Source: CAD feature listing. Evaluate the final solid. Frame: model axes, mm. Coordinates: 2 decimals unless noted, no trailing zeros. Order: outer loops, then holes, each group sorted by start corner. A loop starts at its lowest first (then second) coordinate and runs counter-clockwise, first axis right, second up.
```python
from build123d import *

# Parameters (mm, degrees)
SKETCH1_W           = 339.05
SKETCH1_H           = 130
BOSS_EXTRUDE1_DEPTH = 3.175
SKETCH2_W           = 40
SKETCH2_H           = 3.175
SKETCH2_W_2         = 3.175
SKETCH2_H_2         = 30
CUT_EXTRUDE1_DEPTH  = 10
SKETCH3_W           = 40
SKETCH3_H           = 3.175
CUT_EXTRUDE2_DEPTH  = 364.132184094
LPATTERN1_COUNT     = 3
LPATTERN1_PITCH     = 106.35


with BuildPart() as part:
    # Sketch1 → Boss-Extrude1 (new body)
    with BuildSketch(Plane(origin=(0, 0, 0), x_dir=(0, 0, -1), z_dir=(1, 0, 0))):
        with Locations((169.525, -65)):
            Rectangle(SKETCH1_W, SKETCH1_H)
    extrude(amount=BOSS_EXTRUDE1_DEPTH)

    # Sketch2 → Cut-Extrude1 (cut)
    with BuildSketch(Plane(origin=(3.175, 0, 0), x_dir=(0, 0, -1), z_dir=(1, 0, 0))):
        with Locations((63.175, -11.5875)):
            Rectangle(SKETCH2_W, SKETCH2_H)
        with Locations((169.525, -11.5875)):
            Rectangle(SKETCH2_W, SKETCH2_H)
        with Locations((275.875, -11.5875)):
            Rectangle(SKETCH2_W, SKETCH2_H)
        with Locations((337.4625, -35)):
            Rectangle(SKETCH2_W_2, SKETCH2_H_2)
        with Locations((337.4625, -95)):
            Rectangle(SKETCH2_W_2, SKETCH2_H_2)
        with Locations((1.5875, -35)):
            Rectangle(SKETCH2_W_2, SKETCH2_H_2)
        with Locations((1.5875, -95)):
            Rectangle(SKETCH2_W_2, SKETCH2_H_2)
    extrude(amount=-CUT_EXTRUDE1_DEPTH, mode=Mode.SUBTRACT)

    # Sketch3 → Cut-Extrude2 (cut, through all)
    with BuildSketch(Plane(origin=(3.175, 0, 0), x_dir=(0, 0, -1), z_dir=(1, 0, 0))):
        with Locations((63.18, -128.4125)):
            Rectangle(SKETCH3_W, SKETCH3_H)
    cut_extrude2 = extrude(amount=-CUT_EXTRUDE2_DEPTH, mode=Mode.SUBTRACT)

    # LPattern1: Cut-Extrude2 ×3
    with Locations(*[(0, 0, -i * LPATTERN1_PITCH) for i in range(1, LPATTERN1_COUNT)]):
        add(cut_extrude2, mode=Mode.SUBTRACT)


solid = part.part
```
1. Ray query, line 1 (Y direction, x = 3, z = -50.5) (3 decimals); line 2 (Z direction, x = 1.1, y = -102) (3 decimals). Return the intervals inside material, ascending.
Findings:
line 1: y = -126.825 to -13.175, -10 to 0
line 2: z = -335.875 to -3.175
2. Section query B-B on x = 0.55. Count the separate pieces of the cut face and the enclosed holes in it, plus the area to 3 significant figures.
Findings:
separate pieces: 1
enclosed holes: 3
area: 42,900 mm2
3. Section query A-A on z = -263.5. Return loops of the section in (x, y) (3 decimals).
Findings:
outline: (0, -126.825) - (3.175, -126.825) - (3.175, -13.175) - (0, -13.175) - close; (0, -10) - (3.175, -10) - (3.175, 0) - (0, 0) - close
4. Section query C-C on y = -92.5. Return loops of the section in (x, z) (3 decimals), plus the area to 3 significant figures.
Findings:
outline: (0, -335.875) - (3.175, -335.875) - (3.175, -3.175) - (0, -3.175) - close
area: 1,060 mm2
5. Pin query (flat end, axial travel): P1, Ø1, axis at x = 2, z = -69, coming from the -Y side (3 decimals); P2, Ø1, axis at x = 2, y = -94.5, coming from the +Z side (3 decimals); P3, Ø1.6, axis at x = 2, y = -29.5, coming from the -Z side (3 decimals). Return the tip coordinate at first contact, or that it passes through.
Findings:
P1: stops at y = -126.825
P2: stops at z = -3.175
P3: stops at z = -335.875
